Model file for the job. Use its own axes, mm. A direction names the side the tool comes from. Round coordinates to 2 decimals unless told otherwise and drop trailing zeros. Order: outer loops, then holes, each group sorted by start corner. A loop starts at its lowest first (then second) coordinate and runs counter-clockwise, first axis right, second up. Notation, with made-up numbers: (42.25, 63.25) -> (83.25, 63.25) arc R19 cw to (83.25, 76.25) -> close; hole circle Ø8 at (-16, -2). An arc over 180 degrees is marked (long way). Use CSV: the item, a comma, the result in double quotes.
```python
from build123d import *

# Parameters (mm, degrees)
SKETCH1_W            = 76.2
SKETCH1_H            = 50.8
BOSS_EXTRUDE1_DEPTH  = 1.999996
SKETCH2_W            = 13.999972
SKETCH2_H            = 13.999972
CUT_EXTRUDE1_DEPTH   = 92.668314788
SKETCH3_W            = 4.998974
SKETCH3_H            = 1.307084
CUT_EXTRUDE2_DEPTH   = 2.500122
LPATTERN1_COUNT      = 3
LPATTERN1_PITCH      = 19.048984
LPATTERN1_COUNT_DIR2 = 2
LPATTERN1_PITCH_DIR2 = 19.048984
BOSS_EXTRUDE2_DEPTH  = 76.2
FILLET1_R            = 0.79375


with BuildPart() as part:
    # Sketch1 → Boss-Extrude1 (new, symmetric)
    with BuildSketch(Plane(origin=(0, 0, 0), x_dir=(1, 0, 0), z_dir=(0, 1, 0))):
        with Locations((38.1, 25.4)):
            Rectangle(SKETCH1_W, SKETCH1_H)
    extrude(amount=BOSS_EXTRUDE1_DEPTH, both=True)

    # Sketch2 → Cut-Extrude1 (cut, symmetric)
    with BuildSketch(Plane(origin=(0, 1.999996, 0), x_dir=(1, 0, 0), z_dir=(0, 1, 0))):
        with Locations((19.051016, 34.924492)):
            Rectangle(SKETCH2_W, SKETCH2_H)
    cut_extrude1 = extrude(amount=CUT_EXTRUDE1_DEPTH, both=True, mode=Mode.SUBTRACT)

    # Sketch3 → Cut-Extrude2 (cut)
    with BuildSketch(Plane(origin=(0, 1.999996, 0), x_dir=(1, 0, 0), z_dir=(0, 1, 0))):
        with Locations((19.051016, 42.57802)):
            Rectangle(SKETCH3_W, SKETCH3_H)
        with Locations((19.051016, 27.270964)):
            Rectangle(SKETCH3_W, SKETCH3_H)
    cut_extrude2 = extrude(amount=-CUT_EXTRUDE2_DEPTH, mode=Mode.SUBTRACT)

    # LPattern1: Cut-Extrude1, Cut-Extrude2 3 × 2
    with Locations(*[(i * LPATTERN1_PITCH, 0, j * LPATTERN1_PITCH_DIR2) for i in range(LPATTERN1_COUNT) for j in range(LPATTERN1_COUNT_DIR2) if (i, j) != (0, 0)]):
        add(cut_extrude1, mode=Mode.SUBTRACT)
        add(cut_extrude2, mode=Mode.SUBTRACT)

    # Sketch4 → Boss-Extrude2 (add)
    with BuildSketch(Plane.ZY):
        Polygon((0, -1.999996), (6.928189374, 1.999996), (0, 1.999996), align=None)
    extrude(amount=-BOSS_EXTRUDE2_DEPTH)

    # Fillet1
    fillet1_edges = [part.edges().sort_by_distance(p)[0] for p in [
        (38.1, 1.999996, 6.928189374),
    ]]
    fillet(fillet1_edges, radius=FILLET1_R)


solid = part.part
```
Q1. Cut at C-C (x = 70.5). Give the cut face in (y, z), plus the area to 3 significant figures.
From the geometry:
outline,"(-2, -50.8) -> (2, -50.8) -> (2, 3.97) arc R0.79 ccw to (0.52, 4.36) -> (-2, 0) -> close"
area,"216 mm²"
Q2. Mould opens along X. For faces 1 (the flat face through (64.149, 0, -16)), 2 (the flat face through (0, 0, -23)), 3 (the flat face through (37.57, -0.76, 2.15)) say: +X half, -X half, draft (parallel to the pull), parting line (faces both ways), or undercut.
From the geometry:
face 1,"undercut"
face 2,"-X half"
face 3,"draft"
Q3. Cut at B-B (x = 33.5). Give the cut face in (y, z), plus the area to 3 significant figures.
From the geometry:
outline,"(-2, -50.8) -> (2, -50.8) -> (2, -41.92) -> (-2, -41.92) -> close; (-2, -27.92) -> (2, -27.92) -> (2, -22.88) -> (-2, -22.88) -> close; (-2, -8.88) -> (2, -8.88) -> (2, 3.97) arc R0.79 ccw to (0.52, 4.36) -> (-2, 0) -> close"
area,"104 mm²"
Q4. Cut at D-D (y = -1.2). Give the cut face in (x, z).
From the geometry:
outline,"(0, -50.8) -> (76.2, -50.8) -> (76.2, 1.39) -> (0, 1.39) -> close; hole (12.05, -41.92) -> (26.05, -41.92) -> (26.05, -27.92) -> (12.05, -27.92) -> close; hole (12.05, -22.88) -> (26.05, -22.88) -> (26.05, -8.88) -> (12.05, -8.88) -> close; hole (31.1, -41.92) -> (45.1, -41.92) -> (45.1, -27.92) -> (31.1, -27.92) -> close; hole (31.1, -22.88) -> (45.1, -22.88) -> (45.1, -8.88) -> (31.1, -8.88) -> close; hole (50.15, -41.92) -> (64.15, -41.92) -> (64.15, -27.92) -> (50.15, -27.92) -> close; hole (50.15, -22.88) -> (64.15, -22.88) -> (64.15, -8.88) -> (50.15, -8.88) -> close"
Q5. Cut at A-A (z = -34.5). Give the cut face in (x, y), plus the area to 3 significant figures.
From the geometry:
outline,"(0, -2) -> (12.05, -2) -> (12.05, 2) -> (0, 2) -> close; (26.05, -2) -> (31.1, -2) -> (31.1, 2) -> (26.05, 2) -> close; (45.1, -2) -> (50.15, -2) -> (50.15, 2) -> (45.1, 2) -> close; (64.15, -2) -> (76.2, -2) -> (76.2, 2) -> (64.15, 2) -> close"
area,"137 mm²"
Q6. Which spindle directions (+Z, -Z, +X, -X, +Y, -Y) get a long thin tool onto all of the face, cutting with end or side? Do faces 4 (the flat face through (19, 1, -43.232)), 5 (the flat face through (38, 0, -50.8)), 6 (the flat face through (19, -1, -41.924)). Say none if no direction does.
From the geometry:
face 4,"+Y"
face 5,"-Z, +X, -X, +Y, -Y"
face 6,"+Y, -Y"
Q7. Probe line 1 along X through (y, z) = (-0.1, -42); line 2 along X through (y, z) = (0.65, -15.5); line 3 along Z through (x, y) = (44.5, -1.1). List the from-to ranges inside material, lowest first.
From the geometry:
line 1,"x = 0 to 16.55, 21.55 to 35.6, 40.6 to 54.65, 59.65 to 76.2"
line 2,"x = 0 to 12.05, 26.05 to 31.1, 45.1 to 50.15, 64.15 to 76.2"
line 3,"z = -50.8 to -41.92, -27.92 to -22.88, -8.88 to 1.56"
Q8. Pin check, flat tips, straight feed: pin 1 (0.7 mm diameter, centred on x = 20, z = -42.5, fed in from +Y); pin 2 (1 mm diameter, centred on x = 54.5, y = 0.5, fed in from +Z); pin 3 (1.3 mm diameter, centred on x = 20, y = 0.5, fed in from +Z). Stop position of each tip, or through.
From the geometry:
pin 1,"stops at y = -0.5"
pin 2,"stops at z = 4.73"
pin 3,"stops at z = 4.76"
